from build123d import *

# Parameters (mm, degrees)
SKETCH1_R           = 115.5
SKETCH1_R_2         = 35.5
BOSS_EXTRUDE1_DEPTH = 12.7
SKETCH2_W           = 10
SKETCH2_H           = 63.5
BOSS_EXTRUDE2_DEPTH = 101.6
FILLET1_RADIUS      = 31.75
FILLET1_LENGTH      = 10
FILLET2_RADIUS      = 31.75
FILLET2_LENGTH      = 10
SKETCH3_R           = 11
CUT_EXTRUDE1_DEPTH  = 101.6


with BuildPart() as part:
    # Sketch1 → Boss-Extrude1 (new body)
    with BuildSketch(Plane(origin=(0, 0, 0), x_dir=(1, 0, 0), z_dir=(0, 1, 0))):
        with Locations(Location((0, 0, 0), (0, 0, 270))):
            Circle(SKETCH1_R)
        with Locations(Location((0, 0, 0), (0, 0, 270))):
            Circle(SKETCH1_R_2, mode=Mode.SUBTRACT)
    extrude(amount=BOSS_EXTRUDE1_DEPTH)

    # Sketch2 → Boss-Extrude2 (add)
    with BuildSketch(Plane(origin=(0, 12.7, 0), x_dir=(1, 0, 0), z_dir=(0, 1, 0))):
        with Locations((35.48, 0)):
            Rectangle(SKETCH2_W, SKETCH2_H)
        with Locations((-35.48, 0)):
            Rectangle(SKETCH2_W, SKETCH2_H)
    extrude(amount=BOSS_EXTRUDE2_DEPTH)

    # Fillet1: full round fillet: the end face becomes a half cylinder, R = half its width
    fillet1_face = Plane((35.48, 114.3, 0), x_dir=(1, 0, 0), z_dir=(0, 1, 0))  # on the end face: x along it, z out of the body
    fillet1_slab = fillet1_face.offset(-FILLET1_RADIUS / 2) * Box(FILLET1_LENGTH, 2 * FILLET1_RADIUS, FILLET1_RADIUS, mode=Mode.PRIVATE)  # the body's end, R deep
    fillet1_round = Plane((35.48, 82.55, 0), x_dir=(0, 1, 0), z_dir=(1, 0, 0)) * Cylinder(FILLET1_RADIUS, FILLET1_LENGTH, mode=Mode.PRIVATE)  # its axis R under the face
    add(fillet1_slab - fillet1_round, mode=Mode.SUBTRACT)

    # Fillet2: full round fillet: the end face becomes a half cylinder, R = half its width
    fillet2_face = Plane((-35.48, 114.3, 0), x_dir=(1, 0, 0), z_dir=(0, 1, 0))  # on the end face: x along it, z out of the body
    fillet2_slab = fillet2_face.offset(-FILLET2_RADIUS / 2) * Box(FILLET2_LENGTH, 2 * FILLET2_RADIUS, FILLET2_RADIUS, mode=Mode.PRIVATE)  # the body's end, R deep
    fillet2_round = Plane((-35.48, 82.55, 0), x_dir=(0, 1, 0), z_dir=(1, 0, 0)) * Cylinder(FILLET2_RADIUS, FILLET2_LENGTH, mode=Mode.PRIVATE)  # its axis R under the face
    add(fillet2_slab - fillet2_round, mode=Mode.SUBTRACT)

    # Sketch3 → Cut-Extrude1 (cut)
    with BuildSketch(Plane.ZY.offset(40.48)):
        with Locations((0, 82.55)):
            Circle(SKETCH3_R)
    extrude(amount=-CUT_EXTRUDE1_DEPTH, mode=Mode.SUBTRACT)


solid = part.part
Geometry check sheet. Reference: the model listing, model coordinates, mm. A direction names the side the tool comes from. Round coordinates to 2 decimals unless told otherwise and drop trailing zeros. Write each loop counter-clockwise with the first axis right and the second up, starting at its lowest first coordinate (ties: lowest second). Pieces come first, ordered by that corner, then holes. Notation, with made-up numbers: (63.5, 33.5) - (71.5, 33.5) arc R31 cw to (71.5, 60.5) - close; hole circle Ø8 at (54.25, 37.5). An arc over 180 degrees is marked (long way). One line per item, written item: value.
1. Depth check by flat-ended pin: pin 1 Ø5 at (x, z) = (31, -28.5) entering from +Y; pin 2 Ø2.5 at (x, z) = (34, -2) entering from -Y; pin 3 Ø5 at (x, y) = (-35, 42.5) entering from -Z. Enter the tip coordinate at first touch or a pass-through.
The answers:
pin 1: stops at y = 100.77
pin 2: stops at y = 12.7
pin 3: stops at z = -31.75
2. Cross-section at D-D on x = -84. Record the boundary of the cut face in (y, z), and give its area (3 significant figures).
The answers:
outline: (0, -79.27) - (12.7, -79.27) - (12.7, 79.27) - (0, 79.27) - close
area: 2,010 mm^2
3. Cross-section at B-B on x = 0. Record the boundary of the cut face in (y, z), and give its area (3 significant figures).
The answers:
outline: (0, -115.5) - (12.7, -115.5) - (12.7, -35.5) - (0, -35.5) - close; (0, 35.5) - (12.7, 35.5) - (12.7, 115.5) - (0, 115.5) - close
area: 2,030 mm^2
4. Cross-section at C-C on y = 67. Record the boundary of the cut face in (x, z).
The answers:
outline: (-40.48, -31.75) - (-30.48, -31.75) - (-30.48, 31.75) - (-40.48, 31.75) - close; (30.48, -31.75) - (40.48, -31.75) - (40.48, 31.75) - (30.48, 31.75) - close
5. Cross-section at A-A on z = 0. Record the boundary of the cut face in (x, y), and give its area (3 significant figures).
The answers:
outline: (-115.5, 0) - (-35.5, 0) - (-35.5, 12.7) - (-30.48, 12.7) - (-30.48, 71.55) - (-40.48, 71.55) - (-40.48, 12.7) - (-115.5, 12.7) - close; (-40.48, 93.55) - (-30.48, 93.55) - (-30.48, 114.3) - (-40.48, 114.3) - close; (30.48, 12.7) - (35.5, 12.7) - (35.5, 0) - (115.5, 0) - (115.5, 12.7) - (40.48, 12.7) - (40.48, 71.55) - (30.48, 71.55) - close; (30.48, 93.55) - (40.48, 93.55) - (40.48, 114.3) - (30.48, 114.3) - close
area: 3,620 mm^2
6. Scan lines: L1, parallel to X at y = 61, z = -19.5; L2, parallel to Z at x = -37, y = 82; L3, parallel to X at y = 4.5, z = 0. Record each from-to range of solid material in increasing order.
The answers:
L1: x = -40.48 to -30.48, 30.48 to 40.48
L2: z = -31.75 to -10.99, 10.99 to 31.75
L3: x = -115.5 to -35.5, 35.5 to 115.5
7. Set-up check for faces 5 (the face through (40.48, 63, 0)), 6 (the face through (30.48, 63, 0)), 7 (the face through (-36, 47, -31.75)), 8 (the face through (-36, 47, 31.75)): record each of +Z, -Z, +X, -X, +Y, -Y from which the full face is reachable in a straight line by a thin tool's end or side.
The answers:
face 5: +Z, -Z, +X, +Y
face 6: +Z, -Z, +Y
face 7: -Z, +X, -X, +Y
face 8: +Z, +X, -X, +Y
8. Mould release check, pull along Z, two halves, no side actions. Record for faces 1 (the face through (-31.495, 6.261, 16.381)), 2 (the face through (35.55, 114.292, -0.698)), 3 (the face through (27, 0, 24)), 4 (the face through (35, 47, -31.75)): released by +Z, released by -Z, zero draft, split by the parting line, or undercut.
The answers:
face 1: undercut
face 2: split by the parting line
face 3: zero draft
face 4: released by -Z
